The listing builds one solid part. Answer for the finished solid, in the listing's coordinates (mm). Face numbers are marked on the shaded views. A direction names the side the tool comes from. Round coordinates to 2 decimals unless told otherwise and drop trailing zeros. Write each loop counter-clockwise with the first axis right and the second up, starting at its lowest first coordinate (ties: lowest second). Pieces come first, ordered by that corner, then holes.
Item 1: A tool of negligible diameter and unlimited length cuts with its end or side. For the marked faces 4 and 5, from which of +Z, -Z, +X, -X, +Y, -Y can it reach the whole face along a straight path? Write none if from no direction.
Item 2: Find the intervals of material crossed by probe 1 along Y at (x, z) = (10, 7); probe 2 along Z at (x, y) = (19, 5); probe 3 along Z at (x, y) = (18, -22.75), in increasing order.
Item 3: For a pull along Y with two mould halves and no side action, classify the marked faces 1, 2 and 3 as +Y half, -Y half, draft (parallel to the pull), parting line (faces both ways), or undercut.
Item 4: Each of these flat-tipped pins is pushed along its axis until it touches: pin 1 (3 mm diameter, centred on x = 12, z = 63, fed in from -Y); pin 2 (1.5 mm diameter, centred on x = 6.5, z = 76, fed in from -Y); pin 3 (6 mm diameter, centred on x = 5.5, y = 4, fed in from -Z); pin 4 (3.5 mm diameter, centred on x = 18, z = 44.23, fed in from +Y). Where does it stop, or does it pass through?
Item 5: Find section A-A on x = 13.25. Give the vertices of the cut face in (y, z).
Item 6: Find section B-B on z = 24.5. Give the vertices of the cut face in (x, y), then the cut area to 3 significant figures.
```python
from build123d import *

# Parameters (mm, degrees)
F1_DEPTH        = 25
F2_R            = 7
F3_R            = 5
F4_R            = 10
F5_R            = 5
F6_R            = 10
F7_R            = 10
F8_R            = 1
F9_R            = 5
F10_R           = 1
F12_D           = 4
F12_CSINK_D     = 7
F12_CSINK_ANGLE = 90


with BuildPart() as f1:
    # F0 (on Right) → F1 (new body)
    with BuildSketch(Plane.YZ):
        Polygon((-25, 60), (-25, 0), (0, 0), (10.606602, 10.606602), (7.071068, 14.142136), (-1.812448, 5.25862), (-20, 5.25862), (-20, 57.113249), (46.782032, 95.669873), (44.282032, 100), align=None)
    extrude(amount=F1_DEPTH)

    # F2
    f2_edges = [f1.edges().sort_by_distance(p)[0] for p in [
        (25, 8.838835, 12.374369),
        (0, 8.838835, 12.374369),
        (25, 45.532032, 97.834936),
        (0, 45.532032, 97.834936),
    ]]
    fillet(f2_edges, radius=F2_R)

    # F3
    f3_edges = [f1.edges().sort_by_distance(p)[0] for p in [
        (12.5, -20, 57.113249),
    ]]
    fillet(f3_edges, radius=F3_R)

    # F4
    f4_edges = [f1.edges().sort_by_distance(p)[0] for p in [
        (12.5, -25, 60),
    ]]
    fillet(f4_edges, radius=F4_R)

    # F5
    f5_edges = [f1.edges().sort_by_distance(p)[0] for p in [
        (12.5, -1.812448, 5.25862),
    ]]
    fillet(f5_edges, radius=F5_R)

    # F6
    f6_edges = [f1.edges().sort_by_distance(p)[0] for p in [
        (12.5, -25, 0),
    ]]
    fillet(f6_edges, radius=F6_R)

    # F7
    f7_edges = [f1.edges().sort_by_distance(p)[0] for p in [
        (12.5, 0, 0),
    ]]
    fillet(f7_edges, radius=F7_R)

    # F8
    f8_edges = [f1.edges().sort_by_distance(p)[0] for p in [
        (0, -25, 32.113249),
    ]]
    fillet(f8_edges, radius=F8_R)

    # F9
    f9_edges = [f1.edges().sort_by_distance(p)[0] for p in [
        (12.5, -20, 5.25862),
    ]]
    fillet(f9_edges, radius=F9_R)

    # F10
    f10_edges = [f1.edges().sort_by_distance(p)[0] for p in [
        (25, -20, 32.242559),
    ]]
    fillet(f10_edges, radius=F10_R)

    # F12 (through all)
    with Locations(Plane(origin=(0, -20, 0), x_dir=(-1, 0, 0), z_dir=(0, 1, 0))):
        with Locations((-18, 44.226497), (-7, 30.25862)):
            CounterSinkHole(F12_D / 2, F12_CSINK_D / 2, counter_sink_angle=F12_CSINK_ANGLE)


solid = f1.part
```
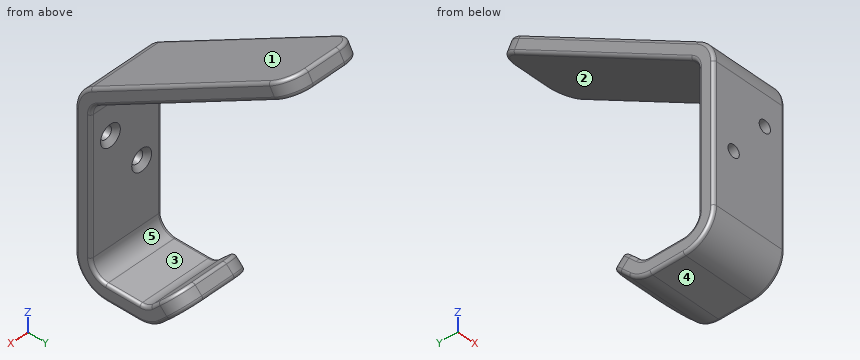
Check values:
1. face 4: -Z, +X, -X, +Y, -Y
1. face 5: +X, -X
2. probe 1: y = -24.54 to -18.79, -0.07 to 7
2. probe 2: z = 5 to 12.07, 71.55 to 77.32
2. probe 3: z = 3.68 to 42.23, 46.23 to 60.55
3. face 1: -Y half
3. face 2: +Y half
3. face 3: undercut
4. pin 1: stops at y = -21.86
4. pin 2: stops at y = 1.41
4. pin 3: stops at z = 1.42
4. pin 4: passes through
5. outline: (-25, 10) arc R10 ccw to (-15, 0) - (-4.14, 0) arc R10 ccw to (2.93, 2.93) - (9.9, 9.9) arc R1 ccw to (9.9, 11.31) - (7.78, 13.44) arc R1 ccw to (6.36, 13.44) - (-0.35, 6.72) arc R5 cw to (-3.88, 5.26) - (-15, 5.26) arc R5 cw to (-20, 10.26) - (-20, 54.23) arc R5 cw to (-17.5, 58.56) - (45.92, 95.17) arc R1 ccw to (46.28, 96.54) - (44.78, 99.13) arc R1 ccw to (43.42, 99.5) - (-20, 62.89) arc R10 ccw to (-25, 54.23) - close
6. outline: (0, -24) arc R1 ccw to (1, -25) - (24, -25) arc R1 ccw to (25, -24) - (25, -21) arc R1 ccw to (24, -20) - (1, -20) arc R1 ccw to (0, -21) - close
6. area: 124 mm2
